Read the model definition and answer for the solid it produces. Units are mm, in the model's axes. A direction names the side the tool comes from. Round coordinates to 2 decimals unless told otherwise and drop trailing zeros. Order: outer loops, then holes, each group sorted by start corner. A loop starts at its lowest first (then second) coordinate and runs counter-clockwise, first axis right, second up.
from build123d import *

# Parameters (mm, degrees)
SKETCH1_W           = 40.5
SKETCH1_H           = 20
BOSS_EXTRUDE1_DEPTH = 37
SKETCH2_W           = 19.6
SKETCH2_H           = 2.7
BOSS_EXTRUDE2_DEPTH = 7.2
CUT_EXTRUDE1_DEPTH  = 43.379151714
BOSS_EXTRUDE3_DEPTH = 2
SKETCH6_R           = 6.5
BOSS_EXTRUDE4_DEPTH = 1.2
SKETCH7_R           = 5.4
BOSS_EXTRUDE5_DEPTH = 0.6
SKETCH8_R           = 3
SKETCH8_R_2         = 2.6
CUT_EXTRUDE2_DEPTH  = 0.6
BOSS_EXTRUDE6_START = 1
SKETCH9_R           = 2.6
BOSS_EXTRUDE6_DEPTH = 1
BOSS_EXTRUDE7_START = 3.2
SKETCH10_R          = 3
BOSS_EXTRUDE7_DEPTH = 3.2
SKETCH11_R          = 1.25
CUT_EXTRUDE3_DEPTH  = 10
SKETCH12_W          = 10.6
SKETCH12_H          = 15.6
BOSS_EXTRUDE8_DEPTH = 0.5
CHAMFER1_SIZE       = 1.6
SKETCH13_W          = 7
SKETCH13_H          = 4
BOSS_EXTRUDE9_DEPTH = 5.2
DRAFT1_ANGLE        = 10


with BuildPart() as part:
    # Sketch1 → Boss-Extrude1 (new body)
    with BuildSketch(Plane(origin=(0, 0, 0), x_dir=(1, 0, 0), z_dir=(0, 1, 0))):
        Rectangle(SKETCH1_W, SKETCH1_H)
    extrude(amount=BOSS_EXTRUDE1_DEPTH)

    # Sketch2 → Boss-Extrude2 (add)
    with BuildSketch(Plane.ZY.offset(20.25)):
        with Locations((0, 29.35)):
            Rectangle(SKETCH2_W, SKETCH2_H)
    boss_extrude2 = extrude(amount=BOSS_EXTRUDE2_DEPTH)

    # Sketch3 → Cut-Extrude1 (cut, through all)
    with BuildSketch(Plane(origin=(0, 30.7, 0), x_dir=(1, 0, 0), z_dir=(0, 1, 0))):
        with BuildLine():
            Line((-27.45, -3.775463215), (-27.45, -6.073333333))
            Line((-27.45, -6.073333333), (-26.121072803, -6.073333333))
            ThreePointArc((-26.121072803, -6.073333333), (-22.218036714, -5.090354029), (-26.022113628, -3.775463215))
            Line((-26.022113628, -3.775463215), (-27.45, -3.775463215))
        make_face()
        with BuildLine():
            Line((-26.121072803, 6.073333333), (-27.45, 6.073333333))
            Line((-27.45, 6.073333333), (-27.45, 3.775463215))
            Line((-27.45, 3.775463215), (-26.022113628, 3.775463215))
            ThreePointArc((-26.022113628, 3.775463215), (-22.218036714, 5.090354029), (-26.121072803, 6.073333333))
        make_face()
    cut_extrude1 = extrude(amount=-CUT_EXTRUDE1_DEPTH, mode=Mode.SUBTRACT)

    # Mirror2: Boss-Extrude2, Cut-Extrude1 across plane
    add(boss_extrude2.mirror(Plane(origin=(0, 0, 0), x_dir=(0, 0, 1), z_dir=(1, 0, 0))))
    add(cut_extrude1.mirror(Plane(origin=(0, 0, 0), x_dir=(0, 0, 1), z_dir=(1, 0, 0))), mode=Mode.SUBTRACT)

    # Sketch5 → Boss-Extrude3 (add)
    with BuildSketch(Plane(origin=(0, 37, 0), x_dir=(1, 0, 0), z_dir=(0, 1, 0))):
        with BuildLine():
            Line((-5.891101056, -9), (14.25, -9))
            Line((14.25, -9), (14.25, -4.8))
            ThreePointArc((14.25, -4.8), (16.65, 0), (14.25, 4.8))
            Line((14.25, 4.8), (14.25, 9))
            Line((14.25, 9), (-5.891101056, 9))
            ThreePointArc((-5.891101056, 9), (-20.25, 0), (-5.891101056, -9))
        make_face()
    extrude(amount=BOSS_EXTRUDE3_DEPTH)

    # Sketch6 → Boss-Extrude4 (add)
    with BuildSketch(Plane(origin=(0, 39, 0), x_dir=(1, 0, 0), z_dir=(0, 1, 0))):
        with Locations(Location((-10.25, 0, 0), (0, 0, 270))):
            Circle(SKETCH6_R)
    extrude(amount=BOSS_EXTRUDE4_DEPTH)

    # Sketch7 → Boss-Extrude5 (add)
    with BuildSketch(Plane(origin=(0, 40.2, 0), x_dir=(1, 0, 0), z_dir=(0, 1, 0))):
        with Locations(Location((-10.25, 0, 0), (0, 0, 270))):
            Circle(SKETCH7_R)
    extrude(amount=BOSS_EXTRUDE5_DEPTH)

    # Sketch8 → Cut-Extrude2 (cut)
    with BuildSketch(Plane(origin=(0, 40.8, 0), x_dir=(1, 0, 0), z_dir=(0, 1, 0))):
        with Locations(Location((-10.25, 0, 0), (0, 0, 270))):
            Circle(SKETCH8_R)
        with Locations(Location((-10.25, 0, 0), (0, 0, 270))):
            Circle(SKETCH8_R_2, mode=Mode.SUBTRACT)
    extrude(amount=-CUT_EXTRUDE2_DEPTH, mode=Mode.SUBTRACT)

    # Sketch9 → Boss-Extrude6 (add)
    with BuildSketch(Plane(origin=(0, 40.8, 0), x_dir=(1, 0, 0), z_dir=(0, 1, 0)).offset(BOSS_EXTRUDE6_START)):
        with Locations(Location((-10.25, 0, 0), (0, 0, 270))):
            Circle(SKETCH9_R)
    extrude(amount=-BOSS_EXTRUDE6_DEPTH)

    # Sketch10 → Boss-Extrude7 (add)
    with BuildSketch(Plane(origin=(0, 41.8, 0), x_dir=(1, 0, 0), z_dir=(0, 1, 0)).offset(BOSS_EXTRUDE7_START)):
        with Locations(Location((-10.25, 0, 0), (0, 0, 270))):
            Circle(SKETCH10_R)
    extrude(amount=-BOSS_EXTRUDE7_DEPTH)

    # Sketch11 → Cut-Extrude3 (cut)
    with BuildSketch(Plane(origin=(0, 45, 0), x_dir=(1, 0, 0), z_dir=(0, 1, 0))):
        with Locations(Location((-10.25, 0, 0), (0, 0, 270))):
            Circle(SKETCH11_R)
    extrude(amount=-CUT_EXTRUDE3_DEPTH, mode=Mode.SUBTRACT)

    # Sketch12 → Boss-Extrude8 (add)
    with BuildSketch(Plane(origin=(0, 39, 0), x_dir=(1, 0, 0), z_dir=(0, 1, 0))):
        with BuildLine():
            Line((14.25, 9), (1.25, 9))
            Line((1.25, 9), (1.25, 2))
            ThreePointArc((1.25, 2), (-0.75, 0), (1.25, -2))
            Line((1.25, -2), (1.25, -9))
            Line((1.25, -9), (14.25, -9))
            Line((14.25, -9), (14.25, 9))
        make_face()
        with Locations((7.75, 0)):
            Rectangle(SKETCH12_W, SKETCH12_H, mode=Mode.SUBTRACT)
    extrude(amount=BOSS_EXTRUDE8_DEPTH)

    # Chamfer1
    chamfer1_edges = [part.edges().sort_by_distance(p)[0] for p in [
        (0, 0, 10),
        (20.25, 0, 0),
        (0, 0, -10),
        (-20.25, 0, 0),
    ]]
    chamfer(chamfer1_edges, length=CHAMFER1_SIZE)

    # Sketch13 → Boss-Extrude9 (add)
    with BuildSketch(Plane.ZY.offset(20.25)):
        with Locations((0, 5.7)):
            Rectangle(SKETCH13_W, SKETCH13_H)
    extrude(amount=BOSS_EXTRUDE9_DEPTH)

    # Draft1
    draft1_faces = [part.faces().sort_by_distance(p)[0] for p in [
        (-22.85, 7.7, 0),
        (-22.85, 5.7, 3.5),
        (-22.85, 5.7, -3.5),
        (-22.85, 3.7, 0),
    ]]
    draft(draft1_faces, Plane(origin=(-20.25, 37, 10), x_dir=(0, 0, -1), z_dir=(-1, 0, 0)), DRAFT1_ANGLE)


solid = part.part
Q1. A cutting plane is placed at B-B, the plane x = 23.5. Give the vertices of the cut face in (y, z), plus the area to 3 significant figures.
Outcome:
outline: (28, -9.8) - (30.7, -9.8) - (30.7, -6.93) - (28, -6.93) - close; (28, -3.07) - (30.7, -3.07) - (30.7, 3.07) - (28, 3.07) - close; (28, 6.93) - (30.7, 6.93) - (30.7, 9.8) - (28, 9.8) - close
area: 32.0 mm2
Q2. A cutting plane is placed at D-D, the plane y = 25. Give the vertices of the cut face in (x, z), plus the area to 3 significant figures.
Outcome:
outline: (-20.25, -10) - (20.25, -10) - (20.25, 10) - (-20.25, 10) - close
area: 810 mm2
Q3. A cutting plane is placed at A-A, the plane x = -21.5. Give the vertices of the cut face in (y, z), plus the area to 3 significant figures.
Outcome:
outline: (3.92, -3.28) - (7.48, -3.28) - (7.48, 3.28) - (3.92, 3.28) - close; (28, -9.8) - (30.7, -9.8) - (30.7, 9.8) - (28, 9.8) - close
area: 76.3 mm2
Q4. A cutting plane is placed at C-C, the plane x = 5. Give the vertices of the cut face in (y, z), plus the area to 3 significant figures.
Outcome:
outline: (0, -8.4) - (1.6, -10) - (37, -10) - (37, -9) - (39.5, -9) - (39.5, -7.8) - (39, -7.8) - (39, 7.8) - (39.5, 7.8) - (39.5, 9) - (37, 9) - (37, 10) - (1.6, 10) - (0, 8.4) - close
area: 775 mm2
Q5. For faces 1 (the face through (-27, 29, -3.775)), 2 (the face through (27, 29, 6.073)), 3 (the face through (-15.04, 40.5, 2.49)), determine the directions among +Z, -Z, +X, -X, +Y, -Y from which every point of the face is accessible in a straight line to the end or side of a thin tool.
Outcome:
face 1: -X, +Y, -Y
face 2: +X, +Y, -Y
face 3: +Y
Q6. Straight lines are drawn through the part: probe 1 along X at (y, z) = (40.4, 0); probe 2 along X at (y, z) = (37.5, 0); probe 3 along X at (y, z) = (42, 0). For each, find the intervals that lie inside material, in ascending order.
Outcome:
probe 1: x = -15.65 to -13.25, -12.85 to -11.5, -9 to -7.65, -7.25 to -4.85
probe 2: x = -20.25 to -11.5, -9 to 16.65
probe 3: x = -13.25 to -11.5, -9 to -7.25
Q7. For a pull along X with two mould halves and no side action, classify faces 4 (the face through (-9, 40, 0)), 5 (the face through (-18, 37, -8)), 6 (the face through (27.45, 29, 8)) as released by +X, released by -X, zero draft, split by the parting line, or undercut.
Outcome:
face 4: undercut
face 5: zero draft
face 6: released by +X
Q8. Flat-ended cylindrical pins translate along their axes: pin 1 (0.8 mm diameter, centred on x = 22.5, y = 29, fed in from -Z); pin 2 (12 mm diameter, centred on y = 7, z = 2, fed in from +X); pin 3 (8 mm diameter, centred on x = -5.5, z = -8, fed in from +Y); pin 4 (4 mm diameter, centred on x = 24.32, z = -5, fed in from -Y). Find the tip coordinate at first contact, or state that the pin passes through.
Outcome:
pin 1: stops at z = -9.8
pin 2: stops at x = 20.25
pin 3: stops at y = 40.8
pin 4: passes through
